The drawing under review shows one solid part. Ordinate dimensions are in mm from its lowest x, y, z. A direction names the side the tool comes from. Give positions to 0.01 mm unless a question says otherwise; leave off trailing zeros. Order: outer loops, then holes, each group sorted by start corner. A loop starts at its lowest first (then second) coordinate and runs counter-clockwise, first axis right, second up. Notation, with made-up numbers: (41, -12.75) - (66, -12.75) arc R14 cw to (66, 1.25) - close; hole circle Ø4 at (-13, 17). An arc over 180 degrees is marked (long way). Use CSV: the item, a comma, the result in double quotes. Start each with the question number.
1. Take a section at B-B, the plane y = 19. State the section outline as (x, z) points.
2. Take a section at A-A, the plane x = 11. State the section outline as (y, z) points.
3. Machinability: for the marked faces 4, 5 and 6, which of the approach directions +Z, -Z, +X, -X, +Y, -Y give a long, thin tool a straight path to every point of the face, cutting with its end or side? Answer none if there is none.
4. For pin 1 (1.5 mm diameter, centred on x = 6.5, z = 8.5, fed in from -Y); pin 2 (4 mm diameter, centred on y = 12.5, z = 12, fed in from +X); pin 3 (4.5 mm diameter, centred on x = 11, y = 3, fed in from -Z); pin 4 (3 mm diameter, centred on x = 11, y = 19, fed in from -Z), all flat-tipped, find the tip position at first contact; note any pin that passes through.
5. Take a section at D-D, the plane z = 8. State the section outline as (x, y) points, then the cut area to 3 significant figures.
6. Take a section at C-C, the plane x = 8.25. State the section outline as (y, z) points.
7. To check wall thickness, follow line 1 (Y direction, x = 11, z = 4.5); line 2 (X direction, y = 10.25, z = 1.75); line 3 (X direction, y = 9.5, z = 1.75). State the ranges of each line that lie inside material, in increasing order. Write a range as [from, to].
8. Draft analysis for pull direction Y (two halves, no side actions). For the marked faces 1, 2 and 3, state which applies: released by +Y, released by -Y, zero draft, split by the parting line, or undercut.
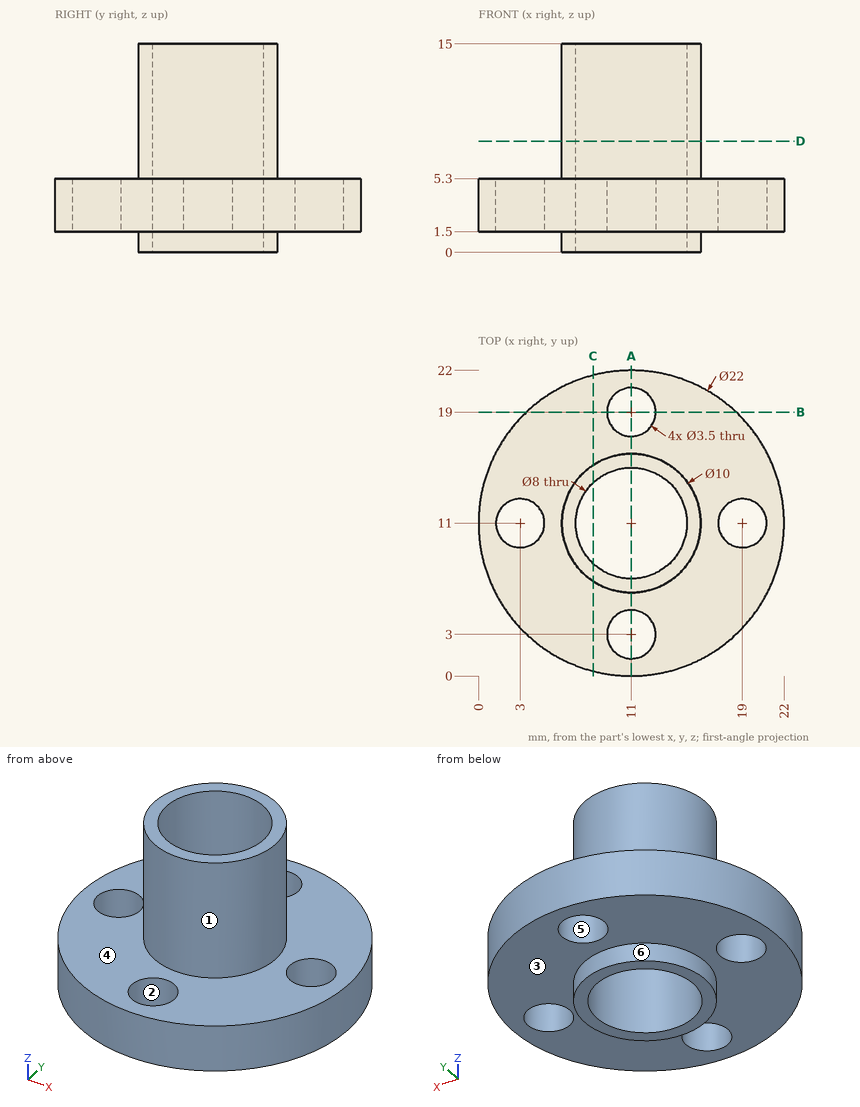
Determined:
1,outline,"(3.45, 1.5) - (9.25, 1.5) - (9.25, 5.3) - (3.45, 5.3) - close; (12.75, 1.5) - (18.55, 1.5) - (18.55, 5.3) - (12.75, 5.3) - close"
2,outline,"(0, 1.5) - (1.25, 1.5) - (1.25, 5.3) - (0, 5.3) - close; (4.75, 1.5) - (6, 1.5) - (6, 0) - (7, 0) - (7, 15) - (6, 15) - (6, 5.3) - (4.75, 5.3) - close; (15, 0) - (16, 0) - (16, 1.5) - (17.25, 1.5) - (17.25, 5.3) - (16, 5.3) - (16, 15) - (15, 15) - close; (20.75, 1.5) - (22, 1.5) - (22, 5.3) - (20.75, 5.3) - close"
3,face 4,"+Z"
3,face 5,"+Z, -Z"
3,face 6,"-Z"
4,pin 1,"stops at y = 7.69"
4,pin 2,"stops at x = 16"
4,pin 3,"stops at z = 1.5"
4,pin 4,"passes through"
5,outline,"circle Ø10 at (11, 11); hole circle Ø8 at (11, 11)"
5,area,"28.3 mm²"
6,outline,"(0.35, 1.5) - (6.82, 1.5) - (6.82, 0) - (8.1, 0) - (8.1, 15) - (6.82, 15) - (6.82, 5.3) - (0.35, 5.3) - close; (13.9, 0) - (15.18, 0) - (15.18, 1.5) - (21.65, 1.5) - (21.65, 5.3) - (15.18, 5.3) - (15.18, 15) - (13.9, 15) - close"
7,line 1,"y = [0, 1.25], [4.75, 7], [15, 17.25], [20.75, 22]"
7,line 2,"x = [0.03, 1.42], [4.58, 7.07], [14.93, 17.42], [20.58, 21.97]"
7,line 3,"x = [0.1, 2.1], [3.9, 7.29], [14.71, 18.1], [19.9, 21.9]"
8,face 1,"split by the parting line"
8,face 2,"undercut"
8,face 3,"zero draft"
